```python
from build123d import *

# Parameters (mm, degrees)
SKETCH1_W                = 40.3
SKETCH1_H                = 20
BOSS_EXTRUDE1_DEPTH      = 36.6
SKETCH5_R                = 10
SKETCH5_R_2              = 3.103657719
SKETCH5_W                = 24.542402665
SKETCH5_H                = 18.960707226
BOSS_EXTRUDE4_DEPTH      = 1
SKETCH7_R                = 8.840936892
BOSS_EXTRUDE5_DEPTH      = 1
BOSS_EXTRUDE7_DEPTH      = 6.65
BOSS_EXTRUDE7_DEPTH_BACK = 46.95
SKETCH8_W                = 18
SKETCH8_H                = 1.536098692
SKETCH10_R               = 3
CUT_EXTRUDE2_DEPTH       = 45.336639532
SKETCH12_R               = 3
CUT_EXTRUDE3_DEPTH       = 45.336639532
SKETCH16_W               = 7
SKETCH16_H               = 3
BOSS_EXTRUDE8_DEPTH      = 5


with BuildPart() as part:
    # Sketch1 → Boss-Extrude1 (new body)
    with BuildSketch(Plane(origin=(0, 0, 0), x_dir=(1, 0, 0), z_dir=(0, 1, 0))):
        with Locations((-5.865266654, 0.347845658)):
            Rectangle(SKETCH1_W, SKETCH1_H)
    extrude(amount=BOSS_EXTRUDE1_DEPTH)

    # Sketch5 → Boss-Extrude4 (add)
    with BuildSketch(Plane(origin=(0, 36.6, 0), x_dir=(1, 0, 0), z_dir=(0, 1, 0))):
        with Locations((4.284733346, 0.347845658)):
            Circle(SKETCH5_R)
        with Locations((-21.934362756, 0.347845658)):
            Circle(SKETCH5_R_2)
        with Locations((-11.108966986, 0.367492045)):
            Rectangle(SKETCH5_W, SKETCH5_H)
    extrude(amount=BOSS_EXTRUDE4_DEPTH)

    # Sketch7 → Boss-Extrude5 (add)
    with BuildSketch(Plane(origin=(0, 37.6, 0), x_dir=(1, 0, 0), z_dir=(0, 1, 0))):
        with Locations(Location((4.284733346, 0.347845658, 0), (0, 0, 90))):
            Circle(SKETCH7_R)
    extrude(amount=BOSS_EXTRUDE5_DEPTH)

    # Sketch8 → Boss-Extrude7 (add, two sides: drawn at the far end of the back side and taken through both)
    with BuildSketch(Plane.ZY.offset(26.015266654).offset(-BOSS_EXTRUDE7_DEPTH_BACK)):
        with Locations((-0.347845658, 27.368049346)):
            Rectangle(SKETCH8_W, SKETCH8_H)
    extrude(amount=BOSS_EXTRUDE7_DEPTH + BOSS_EXTRUDE7_DEPTH_BACK)

    # Sketch10 → Cut-Extrude2 (cut, through all)
    with BuildSketch(Plane(origin=(0, 28.136098692, 0), x_dir=(1, 0, 0), z_dir=(0, 1, 0))):
        with Locations((18.80418216, 4.847845658)):
            Circle(SKETCH10_R)
        with Locations((18.784733346, -4.152133328)):
            Circle(SKETCH10_R)
    extrude(amount=-CUT_EXTRUDE2_DEPTH, mode=Mode.SUBTRACT)

    # Sketch12 → Cut-Extrude3 (cut, through all)
    with BuildSketch(Plane(origin=(0, 28.136098692, 0), x_dir=(1, 0, 0), z_dir=(0, 1, 0))):
        with Locations((-30.515266654, 4.847845658)):
            Circle(SKETCH12_R)
        with Locations((-30.515266654, -4.152154342)):
            Circle(SKETCH12_R)
    extrude(amount=-CUT_EXTRUDE3_DEPTH, mode=Mode.SUBTRACT)

    # Sketch16 → Boss-Extrude8 (add)
    with BuildSketch(Plane.ZY.offset(26.015266654)):
        with Locations((-0.347845658, 5.5)):
            Rectangle(SKETCH16_W, SKETCH16_H)
    extrude(amount=BOSS_EXTRUDE8_DEPTH)


solid = part.part
```
For this review, take the finished solid that the model builds, in its own axes (mm). A direction names the side the tool comes from. Give positions to 0.01 mm unless a question says otherwise; leave off trailing zeros. Write each loop counter-clockwise with the first axis right and the second up, starting at its lowest first coordinate (ties: lowest second). Pieces come first, ordered by that corner, then holes. Notation, with made-up numbers: M 66.25,35.5 L 95.25,35.5 A15 ccw 95.25,61.5 Z; hole C -22,-17 d10. An arc over 180 degrees is marked long. Answer as a JSON object with one key per item and string values. Group by question number.
Item 1: Draft analysis for pull direction Y (two halves, no side actions). For faces 1 (the flat face through (-26.015, 18, 0)), 2 (the flat face through (-6, 18, 9.652)), 3 (the flat face through (17, 28.136, 0)), state which applies: +Y half, -Y half, draft (parallel to the pull), parting line (faces both ways), or undercut.
Item 2: Consider section A-A on x = -14. Write out the cut boundary in (y, z).
Item 3: Consider section B-B on z = -6. Write out the cut boundary in (x, y), plus the area to 3 significant figures.
Item 4: Consider section D-D on x = 10.5. Write out the cut boundary in (y, z).
Item 5: For probe 1 along X at (y, z) = (30, 5.25); probe 2 along Y at (x, z) = (-17, -7); probe 3 along Y at (x, z) = (8, 9.25), list the stretches that pass through material, from the lowest coordinate up. Write a range as [from, to].
Item 6: Tool access review of faces 4 (the flat face through (18, 27, 8.652)), 5 (the flat face through (12, 36.6, 8)), 6 (the flat face through (-29, 27, -9.348)), 7 (the flat face through (12, 36.6, -8)), 8 (the flat face through (-28, 4, 0)): name each direction out of +Z, -Z, +X, -X, +Y, -Y from which nothing blocks a thin tool from reaching the whole face with its end or side.
Item 7: For pin 1 Ø2.5 at (x, z) = (-28, 1) entering from +Y; pin 2 Ø3.5 at (x, y) = (-29, 5.5) entering from +Z; pin 3 Ø6 at (y, z) = (23.5, 3) entering from -X; pin 4 Ø2 at (x, z) = (18, 3) entering from +Y, all flat-tipped, find the tip position at first contact; note any pin that passes through.
Item 8: Consider section C-C on y = 10. Write out the cut boundary in (x, z).
Check result:
{
 "1": {"face 1": "undercut", "face 2": "draft", "face 3": "+Y half"},
 "2": {"outline": "M 0,-10.35 L 36.6,-10.35 L 36.6,-9.85 L 37.6,-9.85 L 37.6,9.11 L 36.6,9.11 L 36.6,9.65 L 0,9.65 Z"},
 "3": {"outline": "M -27.75,26.6 L -26.02,26.6 L -26.02,0 L 14.28,0 L 14.28,26.6 L 16.03,26.6 L 16.03,28.14 L 14.28,28.14 L 14.28,36.6 L 12.53,36.6 L 12.53,37.6 L 11.08,37.6 L 11.08,38.6 L -2.51,38.6 L -2.51,37.6 L -23.38,37.6 L -23.38,36.6 L -26.02,36.6 L -26.02,28.14 L -27.75,28.14 Z", "area": "1,530 mm^2"},
 "4": {"outline": "M 0,-10.35 L 36.6,-10.35 L 36.6,-8.18 L 37.6,-8.18 L 37.6,-6.64 L 38.6,-6.64 L 38.6,5.94 L 37.6,5.94 L 37.6,7.49 L 36.6,7.49 L 36.6,9.65 L 0,9.65 Z"},
 "5": {"probe 1": "x = [-26.02, 14.28]", "probe 2": "y = [0, 37.6]", "probe 3": "y = [0, 36.6]"},
 "6": {"face 4": "+Z, +X, +Y, -Y", "face 5": "+Z, +X, +Y", "face 6": "-Z, -X, +Y, -Y", "face 7": "-Z, +X, +Y", "face 8": "+Z, -Z, -X, -Y"},
 "7": {"pin 1": "stops at y = 28.14", "pin 2": "stops at z = 3.15", "pin 3": "stops at x = -26.02", "pin 4": "passes through"},
 "8": {"outline": "M -26.02,-10.35 L 14.28,-10.35 L 14.28,9.65 L -26.02,9.65 Z"}
}
